from build123d import *

# Parameters (mm, degrees)
F0_W     = 59.06649
F0_H     = 58.101352
F1_DEPTH = 17.018
F2_R     = 10.676277
F3_DEPTH = 16.002
F5_DEPTH = 29.534245
F6_DEPTH = 29.534245


with BuildPart() as f1:
    # F0 (on Top) → F1 (new body)
    with BuildSketch(Plane.XY):
        Rectangle(F0_W, F0_H)
    extrude(amount=F1_DEPTH)

    # F2 (on face) → F3 (join)
    with BuildSketch(Plane.XY.offset(17.018)):
        Circle(F2_R)
    extrude(amount=F3_DEPTH)

    # F4 (on Right) → F5 (cut, through all)
    with BuildSketch(Plane.YZ):
        Polygon((-10.705338, 23.905559), (10.682108, 33.037279), (-10.705338, 33.037279), align=None)
    extrude(amount=-F5_DEPTH, mode=Mode.SUBTRACT)

    # F5_face (on face) → F6 (cut, through all)
    with BuildSketch(Plane(origin=(0, -3.570305, 29.985989), x_dir=(0, 1, 0), z_dir=(-1, 0, 0))):
        Polygon((-7.105972, 6.068022), (-7.105972, -3.034011), (14.211944, -3.034011), align=None)
    extrude(amount=-F6_DEPTH, mode=Mode.SUBTRACT)


solid = f1.part
Model file for the job. Use its own axes, mm. A direction names the side the tool comes from. Give positions to 0.01 mm unless a question says otherwise; leave off trailing zeros. Write each loop counter-clockwise with the first axis right and the second up, starting at its lowest first coordinate (ties: lowest second). Pieces come first, ordered by that corner, then holes. Notation, with made-up numbers: M -11.5,69.25 L -3.5,69.25 A19 ccw -3.5,98.25 Z; hole C 41,28.5 d10. An arc over 180 degrees is marked long. One line per item, written item: value. Start each with the question number.
Q1. Saw through at D-D, the plane x = 19. Write the cut outline in (y, z), plus the area to 3 significant figures.
Q2. Saw through at B-B, the plane x = 2. Write the cut outline in (y, z).
Q3. Drop flat-ended pins along their axis: pin 1 Ø4 at (x, z) = (10, 24) entering from +Y; pin 2 Ø1.5 at (x, y) = (5.5, 14.5) entering from +Z. Give the stop position or say it passes through.
Q4. Saw through at C-C, the plane z = 31. Write the cut outline in (x, y), plus the area to 3 significant figures.
Q5. 3-axis set-ups, long thin cutter, end or side, ignore diameter. For faces 1 (the flat face through (0, 13, 17.018)), 2 (the flat face through (-29.533, 0, 8)): which of +Z, -Z, +X, -X, +Y, -Y reach the whole face in a straight line?
Q6. Probe probe 1 along Z at (x, y) = (-10.5, 9.5); probe 2 along Z at (x, y) = (-3, 0); probe 3 along X at (y, z) = (-8, 19.5). List the from-to ranges inside material, lowest first. Write a range as [from, to].
Q7. Saw through at A-A, the plane y = 23. Write the cut outline in (x, z), plus the area to 3 significant figures.
Output values:
1. outline: M -29.05,0 L 29.05,0 L 29.05,17.02 L -29.05,17.02 Z
1. area: 989 mm²
2. outline: M -29.05,0 L 29.05,0 L 29.05,17.02 L 10.49,17.02 L 10.49,32.95 L -10.49,24 L -10.49,17.02 L -29.05,17.02 Z
3. pin 1: stops at y = 7.07
3. pin 2: stops at z = 17.02
4. outline: M -8.89,5.91 L 8.89,5.91 A10.68 ccw Z
4. area: 59.6 mm²
5. face 1: +Z
5. face 2: +Z, -Z, -X, +Y, -Y
6. probe 1: z = [0, 17.02]
6. probe 2: z = [0, 28.48]
6. probe 3: x = [-7.07, 7.07]
7. outline: M -29.53,0 L 29.53,0 L 29.53,17.02 L -29.53,17.02 Z
7. area: 1,010 mm²
